Can you work these out from the model? Positions are in its coordinate system, mm. Face numbers are marked on the shaded views. Give positions to 0.01 mm unless a question says otherwise; leave off trailing zeros. Write each loop counter-clockwise with the first axis right and the second up, starting at its lowest first coordinate (ties: lowest second). Pieces come first, ordered by that corner, then holes. Notation, with made-up numbers: (13.25, 33.25) - (35.25, 33.25) arc R23 ccw to (35.25, 43.25) - close; hole circle Ø1 at (64, 34). An arc over 180 degrees is marked (long way). Use a Markdown table: item, result. Add a question column.
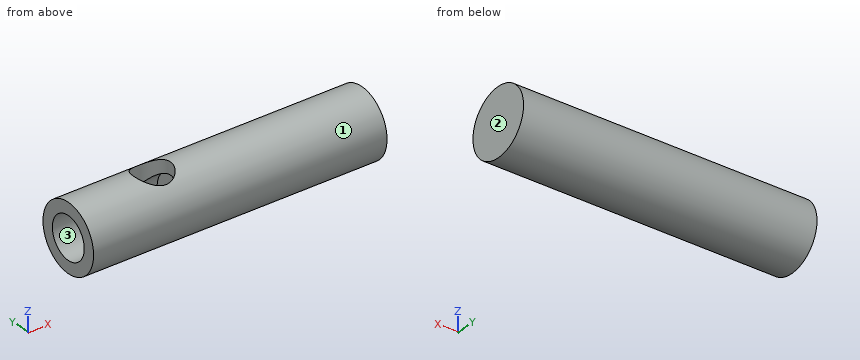
```python
from build123d import *

# Parameters (mm, degrees)
F0_R     = 3.175
F1_DEPTH = 28
F2_R     = 2
F3_DEPTH = 10
F4_R     = 1.75
F5_DEPTH = 3.176


with BuildPart() as f1:
    # F0 (on Right) → F1 (new body)
    with BuildSketch(Plane.YZ):
        Circle(F0_R)
    extrude(amount=F1_DEPTH)

    # F2 (on face) → F3 (cut)
    with BuildSketch(Plane(origin=(0, 0, 0), x_dir=(0, -1, 0), z_dir=(-1, 0, 0))):
        Circle(F2_R)
    extrude(amount=-F3_DEPTH, mode=Mode.SUBTRACT)

    # F4 (on Top) → F5 (cut, through all)
    with BuildSketch(Plane.XY):
        with Locations((8, 0)):
            Circle(F4_R)
    extrude(amount=F5_DEPTH, mode=Mode.SUBTRACT)


solid = f1.part
```
Q1. Suppose I cut it at C-C (x = 11.5). Please give me the cut outline in (y, z) (3 decimals).
Q2. Suppose I cut it at B-B (z = 0). Please give me the cut outline in (x, y) (3 decimals), and give its area (3 significant figures).
Q3. If I drill on probe 1 along Z at (x, y) = (4.75, 0) (3 decimals); probe 2 along X at (y, z) = (-1.5, 1); probe 3 along Y at (x, z) = (8, 2.15), over which ranges is the centre line in solid material (lowest first)? Write a range as [from, to].
Q4. Suppose I cut it at D-D (y = -1.5). Please give me the cut outline in (x, z), and give its area (3 significant figures).
Q5. I'm going to push a flat-ended pin straight in: P1, Ø1, axis at x = 9.5, y = -1, coming from the -Z side. Where does the tip first touch, or does it pass through?
Q6. If we mould it in two halves opening along Y, with no side actions, what happens to the marked faces 1, 2 and 3? For each: released by +Y, released by -Y, zero draft, split by the parting line, or undercut.
Q7. Suppose I cut it at A-A (y = 0). Please give me the cut outline in (x, z) (3 decimals).
Derived:
| question | item | result |
|---|---|---|
| 1 | outline | circle Ø6.35 at (0, 0) |
| 2 | outline | (0, -3.175) - (28, -3.175) - (28, 3.175) - (0, 3.175) - (0, 2) - (10, 2) - (10, -2) - (0, -2) - close |
| 2 | area | 138 mm² |
| 3 | probe 1 | [-3.175, -2], [2, 3.175] |
| 3 | probe 2 | [10, 28] |
| 3 | probe 3 | [-2.34, -1.75], [1.75, 2.34] |
| 4 | outline | (0, -2.8) - (28, -2.8) - (28, 2.8) - (8.9, 2.8) - (8.9, 1.32) - (10, 1.32) - (10, -1.32) - (0, -1.32) - close; (0, 1.32) - (7.1, 1.32) - (7.1, 2.8) - (0, 2.8) - close |
| 4 | area | 128 mm² |
| 5 | P1 | z = -3.14 |
| 6 | face 1 | split by the parting line |
| 6 | face 2 | zero draft |
| 6 | face 3 | undercut |
| 7 | outline | (0, -3.175) - (28, -3.175) - (28, 3.175) - (9.75, 3.175) - (9.75, 2) - (10, 2) - (10, -2) - (0, -2) - close; (0, 2) - (6.25, 2) - (6.25, 3.175) - (0, 3.175) - close |
